```python
from build123d import *

# Parameters (mm, degrees)
REVOLVE1_ANGLE          = 180
SKETCH3_W               = 9
SKETCH3_H               = 120
BOSS_EXTRUDE3_DEPTH     = 3.264935
BOSS_EXTRUDE4_REACH     = 158
SKETCH6_R               = 27
SKETCH6_R_2             = 18
SKETCH7_R               = 18
CUT_EXTRUDE1_DEPTH      = 157
BOSS_EXTRUDE5_DEPTH     = 54
CUT_EXTRUDE2_DEPTH      = 175.0000001
CUT_EXTRUDE2_DEPTH_BACK = 1


with BuildPart() as part:
    # Sketch1 → Revolve1 (revolve)
    with BuildSketch(Plane.XY):
        Polygon((144, 9), (144, 111), (0, 111), (0, 120), (153, 120), (153, 0), (0, 0), (0, 9), align=None)
    revolve(axis=Axis((0, 0, 0), (0, 1, 0)), revolution_arc=REVOLVE1_ANGLE)

    # Sketch3 → Boss-Extrude3 (add)
    with BuildSketch(Plane(origin=(156, 0, 0), x_dir=(0, 0, -1), z_dir=(1, 0, 0))):
        with Locations((4.5, 60)):
            Rectangle(SKETCH3_W, SKETCH3_H)
    boss_extrude3 = extrude(amount=-BOSS_EXTRUDE3_DEPTH)

    # Mirror4: Boss-Extrude3 across plane
    add(boss_extrude3.mirror(Plane(origin=(0, 0, 0), x_dir=(0, 0, 1), z_dir=(1, 0, 0))))

    # Sketch6 → Boss-Extrude4 (add, up to next)
    with BuildSketch(Plane(origin=(0, 0, -156), x_dir=(-1, 0, 0), z_dir=(0, 0, -1)), mode=Mode.PRIVATE) as boss_extrude4_sk1:
        with Locations((0, 60)):
            Circle(SKETCH6_R)
        with Locations((0, 60)):
            Circle(SKETCH6_R_2, mode=Mode.SUBTRACT)
    boss_extrude4_tool1 = extrude(boss_extrude4_sk1.sketch, amount=-BOSS_EXTRUDE4_REACH, mode=Mode.PRIVATE) - part.part
    add(boss_extrude4_tool1.solids().sort_by_distance((26.236325, 60, -156))[0])

    # Sketch7 → Cut-Extrude1 (cut, through all)
    with BuildSketch(Plane(origin=(0, 0, -156), x_dir=(-1, 0, 0), z_dir=(0, 0, -1))):
        with Locations((0, 60)):
            Circle(SKETCH7_R)
    extrude(amount=-CUT_EXTRUDE1_DEPTH, mode=Mode.SUBTRACT)

    # Sketch8 → Boss-Extrude5 (add)
    with BuildSketch(Plane(origin=(0, -54, 0), x_dir=(1, 0, 0), z_dir=(0, 1, 0))):
        with BuildLine():
            Line((78, 0), (27, 0))
            ThreePointArc((27, 0), (0, 27), (-27, 0))
            Line((-27, 0), (-78, 0))
            Line((-78, 0), (-78, 21))
            Line((-78, 21), (-43.16248371, 21))
            ThreePointArc((-43.16248371, 21), (0, 48), (43.16248371, 21))
            Line((43.16248371, 21), (78, 21))
            Line((78, 21), (78, 0))
        make_face()
    boss_extrude5 = extrude(amount=BOSS_EXTRUDE5_DEPTH)

    # Sketch9 → Cut-Extrude2 (cut, two sides)
    with BuildSketch(Plane(origin=(0, -54, 0), x_dir=(1, 0, 0), z_dir=(0, 1, 0))) as cut_extrude2_sk:
        with BuildLine():
            Line((27, -490.936586386), (27, 0))
            ThreePointArc((27, 0), (0, 27), (-27, 0))
            Line((-27, 0), (-27, -490.936586386))
            Line((-27, -490.936586386), (-27, -1472.809759159))
            Line((-27, -1472.809759159), (27, -1472.809759159))
            Line((27, -1472.809759159), (27, -490.936586386))
        make_face()
    extrude(amount=CUT_EXTRUDE2_DEPTH, mode=Mode.SUBTRACT)
    extrude(cut_extrude2_sk.sketch, amount=-CUT_EXTRUDE2_DEPTH_BACK, mode=Mode.SUBTRACT)

    # Mirror6: Boss-Extrude5 across plane
    add(boss_extrude5.mirror(Plane.ZX.offset(60)))


solid = part.part
```
CAD build for the part. Positions are in the model's coordinates, mm. A direction names the side the tool comes from. Round coordinates to 2 decimals unless told otherwise and drop trailing zeros. Order: outer loops, then holes, each group sorted by start corner. A loop starts at its lowest first (then second) coordinate and runs counter-clockwise, first axis right, second up. Notation, with made-up numbers: (5, 68.5) -> (14, 68.5) arc R26 cw to (14, 82.5) -> close; hole circle Ø4 at (1.5, 50.25). An arc over 180 degrees is marked (long way). Write item = value, one per line.
(1) Cut at B-B (y = 60). Write the cut outline in (x, z), plus the area to 3 significant figures.
Answers follow:
outline = (-156, -9) -> (-152.74, -9) arc R153 ccw to (-27, -150.6) -> (-27, -156) -> (-18, -156) -> (-18, -142.87) arc R144 cw to (-144, 0) -> (-156, 0) -> close; (18, -156) -> (27, -156) -> (27, -150.6) arc R153 ccw to (152.74, -9) -> (156, -9) -> (156, 0) -> (144, 0) arc R144 cw to (18, -142.87) -> close
area = 4,010 mm²
(2) Cut at C-C (y = 3.5). Write the cut outline in (x, z).
Answers follow:
outline = (-156, -9) -> (-152.74, -9) arc R153 ccw to (152.74, -9) -> (156, -9) -> (156, 0) -> (27, 0) arc R27 cw to (-27, 0) -> (-156, 0) -> close
(3) Flat gauge pins, fed straight in: P1, Ø5, axis at y = 43, z = -63.5, coming from the -X side; P2, Ø1.6, axis at x = 154, y = 71, coming from the -Z side; P3, Ø10.5, axis at x = 62, y = -35, coming from the -Z side. Where does each tip first touch, or does it go through?
Answers follow:
P1 = -140.31
P2 = -9
P3 = -21
(4) Drill centre lines: L1, parallel to Y at x = 116, z = -67; L2, parallel to X at y = 60, z = -153.05; L3, parallel to Y at x = 0, z = -152.9. Where is each one in solid material? Low to high.
Answers follow:
L1 = 0 to 9, 111 to 120
L2 = -27 to -18, 18 to 27
L3 = 0 to 42, 78 to 120
(5) Pull direction X, two halves, no side cores. Call faces 5 (the flat face through (-78, -27, -10)), 6 (the cylindrical face through (-0.751, 147.378, -47.994)), 7 (the flat face through (-2, 111, -57)): +X half, -X half, draft (parallel to the pull), parting line (faces both ways), or undercut.
Answers follow:
face_5 = -X half
face_6 = parting line
face_7 = undercut
(6) 3-axis set-ups, long thin cutter, end or side, ignore diameter. For faces 1 (the flat face through (-61, -27, -21)), 2 (the cylindrical face through (3.166, 38.047, -143.965)), 3 (the flat face through (78, -27, -11)), 4 (the flat face through (60, -27, -21)): which of +Z, -Z, +X, -X, +Y, -Y reach the whole face in a straight line?
Answers follow:
face_1 = -Z, -X, -Y
face_2 = +Z
face_3 = +Z, -Z, +X, -Y
face_4 = -Z, +X, -Y
(7) Cut at D-D (z = -112). Write the cut outline in (x, y), plus the area to 3 significant figures.
Answers follow:
outline = (-104.24, 0) -> (104.24, 0) -> (104.24, 120) -> (-104.24, 120) -> close; hole (-90.51, 9) -> (90.51, 9) -> (90.51, 111) -> (-90.51, 111) -> close
area = 6,550 mm²
(8) Cut at A-A (x = 0). Write the cut outline in (y, z).
Answers follow:
outline = (-54, -48) -> (0, -48) -> (0, -153) -> (33, -153) -> (33, -156) -> (42, -156) -> (42, -144) -> (9, -144) -> (9, -27) -> (-54, -27) -> close; (78, -156) -> (87, -156) -> (87, -153) -> (120, -153) -> (120, -48) -> (174, -48) -> (174, -27) -> (111, -27) -> (111, -144) -> (78, -144) -> close
